Drawing for the job (mm, zero at the part's lowest x, y, z). A direction names the side the tool comes from. Coordinates: 2 decimals unless noted, no trailing zeros. Write each loop counter-clockwise with the first axis right and the second up, starting at its lowest first coordinate (ties: lowest second). Pieces come first, ordered by that corner, then holes. Notation, with made-up numbers: M 46,-25 L 71,-25 A23 ccw 71,5 Z; hole C 40,-37 d7. An arc over 180 degrees is marked long. Put each result on its own line as item: value. Start each with the question number.
Q1. Cut at C-C (z = 40.5). Write the cut outline in (x, y) (3 decimals).
Q2. Drill centre lines: line 1 along Z through (x, y) = (14, 5.5); line 2 along Y through (x, z) = (68, 31) (3 decimals); line 3 along X through (y, z) = (16.25, 43). Where is each one in solid material? Low to high.
Q3. Cut at D-D (x = 86). Write the cut outline in (y, z) (3 decimals), then the cut area to 3 significant figures.
Q4. Pull direction X, two halves, no side cores. Call the marked faces 1 and 2: pulls with the +X half, pulls with the -X half, needs draft (parallel to the pull), parting line crosses it, or undercut.
Q5. Cut at A-A (x = 71). Write the cut outline in (y, z) (3 decimals), then the cut area to 3 significant figures.
Q6. Cut at B-B (y = 17.5). Write the cut outline in (x, z), then the cut area to 3 significant figures.
Q7. Which spindle directions (+Z, -Z, +X, -X, +Y, -Y) get a long thin tool onto all of the face, cutting with end or side? Do the marked faces 3 and 4. Say none if no direction does.
Q8. Drop flat-ended pins along their axis: pin 1 (3 mm diameter, centred on x = 48.5, y = 6.5, fed in from +Z); pin 2 (3 mm diameter, centred on y = 15, z = 21, fed in from -X); pin 3 (2.5 mm diameter, centred on x = 43, y = 23.5, fed in from +Z). Give the stop position or say it passes through.
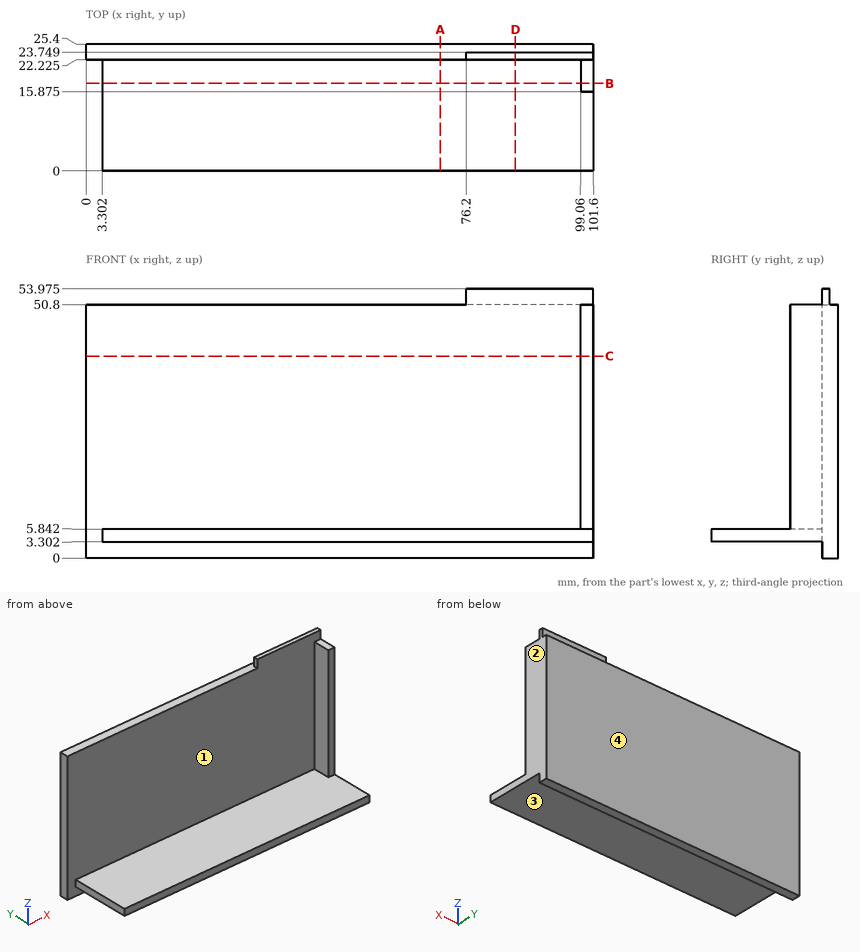
Computed values:
1. outline: M 0,22.225 L 99.06,22.225 L 99.06,15.875 L 101.6,15.875 L 101.6,25.4 L 0,25.4 Z
2. line 1: 3.3 to 5.84
2. line 2: 22.225 to 25.4
2. line 3: 99.06 to 101.6
3. outline: M 0,3.302 L 22.225,3.302 L 22.225,0 L 25.4,0 L 25.4,50.8 L 23.749,50.8 L 23.749,53.975 L 22.225,53.975 L 22.225,5.842 L 0,5.842 Z
3. area: 223 mm2
4. face 1: needs draft
4. face 2: pulls with the +X half
5. outline: M 0,3.302 L 22.225,3.302 L 22.225,0 L 25.4,0 L 25.4,50.8 L 22.225,50.8 L 22.225,5.842 L 0,5.842 Z
5. area: 218 mm2
6. outline: M 3.3,3.3 L 101.6,3.3 L 101.6,50.8 L 99.06,50.8 L 99.06,5.84 L 3.3,5.84 Z
6. area: 364 mm2
7. face 3: -Z, +X, -X, -Y
7. face 4: +Z, -Z, +X, -X, +Y
8. pin 1: z = 5.84
8. pin 2: x = 99.06
8. pin 3: z = 50.8
